Build history of the part. All positions in model axes, mm. Face numbers are marked on the shaded views. Give positions to 0.01 mm unless a question says otherwise; leave off trailing zeros. Order: outer loops, then holes, each group sorted by start corner. A loop starts at its lowest first (then second) coordinate and runs counter-clockwise, first axis right, second up. Notation, with made-up numbers: (-29.75, -12.5) - (18.25, -12.5) arc R20 ccw to (18.25, -4.5) - close; hole circle Ø10 at (18, 79.5). An arc over 180 degrees is marked (long way). One line per item, written item: value.
```python
from build123d import *

# Parameters (mm, degrees)
BOSS_EXTRUDE2_DEPTH = 8
SKETCH2_R           = 3.15
CUT_EXTRUDE1_DEPTH  = 8
BOSS_EXTRUDE4_DEPTH = 2
CUT_EXTRUDE2_DEPTH  = 14
SKETCH5_R           = 2.15
CUT_EXTRUDE3_DEPTH  = 14
SKETCH6_R           = 3.5
CUT_EXTRUDE4_DEPTH  = 2.6
CUT_EXTRUDE5_DEPTH  = 18.5
BOSS_EXTRUDE7_DEPTH = 8
SKETCH9_R           = 3.15
CUT_EXTRUDE6_DEPTH  = 8
CUT_EXTRUDE8_DEPTH  = 8
BOSS_EXTRUDE8_DEPTH = 8
CUT_EXTRUDE9_DEPTH  = 2.5


with BuildPart() as part:
    # Sketch1 → Boss-Extrude2 (new body)
    with BuildSketch(Plane(origin=(0, 0, 0), x_dir=(1, 0, 0), z_dir=(0, 1, 0))):
        Polygon((-36.064195387, 30.19821093), (-36.064195387, 45.055140387), (-24.456215945, 60.508200645), (25.928290152, 75.028423128), (63.192701615, 49.978777876), (57.8600206, 4.654046233), (5.024212079, -12.575443702), (-26.79369062, -0.934399252), align=None)
    extrude(amount=BOSS_EXTRUDE2_DEPTH)

    # Sketch2 → Cut-Extrude1 (cut)
    with BuildSketch(Plane(origin=(0, 8, 0), x_dir=(1, 0, 0), z_dir=(0, 1, 0))):
        with Locations((-0.992606529, 5.023658057)):
            Circle(SKETCH2_R)
        with Locations((-23.973939823, 24.307286348)):
            Circle(SKETCH2_R)
    extrude(amount=-CUT_EXTRUDE1_DEPTH, mode=Mode.SUBTRACT)

    # Sketch3 → Boss-Extrude4 (add)
    with BuildSketch(Plane(origin=(0, 8, 0), x_dir=(1, 0, 0), z_dir=(0, 1, 0))):
        Polygon((-5.747908307, 51.79510143), (2.909877598, 46.790828933), (8.164363719, 55.881504134), (-0.493422186, 60.885776631), align=None)
        Polygon((-2.344608524, 37.700153733), (2.909877598, 46.790828933), (-5.747908307, 51.79510143), (-11.002394429, 42.70442623), align=None)
        Polygon((37.108131922, 27.023952571), (45.765917827, 22.019680074), (51.020403949, 31.110355274), (42.362618044, 36.114627771), align=None)
        Polygon((40.511431705, 12.929004873), (45.765917827, 22.019680074), (37.108131922, 27.023952571), (31.8536458, 17.93327737), align=None)
    extrude(amount=BOSS_EXTRUDE4_DEPTH)

    # Sketch4 → Cut-Extrude2 (cut)
    with BuildSketch(Plane(origin=(0, 8, 0), x_dir=(1, 0, 0), z_dir=(0, 1, 0))):
        Polygon((8.164363719, 55.881504134), (-2.344608524, 37.700153733), (31.8536458, 17.93327737), (42.362618044, 36.114627771), align=None)
    extrude(amount=-CUT_EXTRUDE2_DEPTH, mode=Mode.SUBTRACT)

    # Sketch5 → Cut-Extrude3 (cut)
    with BuildSketch(Plane(origin=(0, 10, 0), x_dir=(1, 0, 0), z_dir=(0, 1, 0))):
        with Locations((-3.921151603, 44.964072229)):
            Circle(SKETCH5_R)
        with Locations((1.083120894, 53.621858134)):
            Circle(SKETCH5_R)
        with Locations((43.939161123, 28.850709275)):
            Circle(SKETCH5_R)
        with Locations((38.934888626, 20.19292337)):
            Circle(SKETCH5_R)
    extrude(amount=-CUT_EXTRUDE3_DEPTH, mode=Mode.SUBTRACT)

    # Sketch6 → Cut-Extrude4 (cut)
    with BuildSketch(Plane.XZ):
        with Locations((43.939161123, -28.850709275)):
            Circle(SKETCH6_R)
        with Locations((38.934888626, -20.19292337)):
            Circle(SKETCH6_R)
        with Locations((1.083120894, -53.621858134)):
            Circle(SKETCH6_R)
        with Locations((-3.921151603, -44.964072229)):
            Circle(SKETCH6_R)
    extrude(amount=-CUT_EXTRUDE4_DEPTH, mode=Mode.SUBTRACT)

    # Sketch7 → Cut-Extrude5 (cut)
    with BuildSketch(Plane(origin=(0, 8, 0), x_dir=(1, 0, 0), z_dir=(0, 1, 0))):
        Polygon((-23.90080129, 101.032848336), (-57.901406204, 20.736967462), (-18.158957139, -32.533824917), (87.924213713, -9.961236853), (85.311975199, 49.315634488), align=None)
        Polygon((-40.820623888, 23.42964982), (-5.371906334, -12.019067733), (42.940552226, -17.400063196), (73.057764711, 41.083606285), (-8.197554073, 82.927487203), align=None, mode=Mode.SUBTRACT)
    extrude(amount=-CUT_EXTRUDE5_DEPTH, mode=Mode.SUBTRACT)

    # Sketch8 → Boss-Extrude7 (add)
    with BuildSketch(Plane(origin=(0, 8, 0), x_dir=(1, 0, 0), z_dir=(0, 1, 0))):
        Polygon((-8.197554073, 82.927487203), (-40.820623888, 23.42964982), (-5.371906334, -12.019067733), (42.940552226, -17.400063196), (73.057764711, 41.083606285), align=None)
        Polygon((7.41963674, 62.005546744), (-9.746922841, 64.747246038), (-32.401642497, 23.42964982), (0, -4.674812176), (46.197479834, 11.841771544), (56.025503799, 35.943618774), align=None, mode=Mode.SUBTRACT)
    extrude(amount=-BOSS_EXTRUDE7_DEPTH)

    # Sketch9 → Cut-Extrude6 (cut)
    with BuildSketch(Plane(origin=(0, 0, 0), x_dir=(-1, 0, 0), z_dir=(0, -1, 0))):
        with Locations((-28.941808693, 3.473889793)):
            Circle(SKETCH9_R)
    extrude(amount=-CUT_EXTRUDE6_DEPTH, mode=Mode.SUBTRACT)

    # Sketch10 → Cut-Extrude8 (cut)
    with BuildSketch(Plane(origin=(0, 8, 0), x_dir=(1, 0, 0), z_dir=(0, 1, 0))):
        Polygon((-51.027907223, 26.499697203), (-18.337970987, 89.979258173), (70.618900133, 64.73001084), (85.862243499, 8.329361683), (41.198193823, -31.646717715), (-23.676019088, -9.814381331), align=None)
        with BuildLine():
            Line((-33.872566493, 31.841833363), (-7.610913822, 63.637460521))
            ThreePointArc((-7.610913822, 63.637460521), (-0.606725689, 67.783190008), (7.431616747, 66.506171896))
            Line((7.431616747, 66.506171896), (48.870452229, 43.677060264))
            ThreePointArc((48.870452229, 43.677060264), (53.514897305, 39.092266426), (55.073012074, 32.754799821))
            Line((55.073012074, 32.754799821), (41.706263242, -9.064889609))
            ThreePointArc((41.706263242, -9.064889609), (33.18888877, -18.343686498), (20.602861854, -17.860296318))
            Line((20.602861854, -17.860296318), (-29.950777497, 7.924950794))
            ThreePointArc((-29.950777497, 7.924950794), (-37.823070784, 18.242703419), (-34.700474084, 30.839465332))
            Line((-34.700474084, 30.839465332), (-33.872566493, 31.841833363))
        make_face(mode=Mode.SUBTRACT)
    extrude(amount=-CUT_EXTRUDE8_DEPTH, mode=Mode.SUBTRACT)

    # Sketch12 → Boss-Extrude8 (add)
    with BuildSketch(Plane(origin=(0, 8, 0), x_dir=(1, 0, 0), z_dir=(0, 1, 0))):
        with BuildLine():
            Line((-34.700474084, 30.839465332), (-23.799416497, 10.878604368))
            Line((-23.799416497, 10.878604368), (16.273254251, -10.775107124))
            Line((16.273254251, -10.775107124), (41.706263242, -9.064889609))
            ThreePointArc((41.706263242, -9.064889609), (33.18888877, -18.343686498), (20.602861854, -17.860296318))
            Line((20.602861854, -17.860296318), (-29.950777497, 7.924950794))
            ThreePointArc((-29.950777497, 7.924950794), (-37.823070784, 18.242703419), (-34.700474084, 30.839465332))
        make_face()
    extrude(amount=-BOSS_EXTRUDE8_DEPTH)

    # Sketch13 → Cut-Extrude9 (cut)
    with BuildSketch(Plane(origin=(0, 10, 0), x_dir=(1, 0, 0), z_dir=(0, 1, 0))):
        Polygon((37.108131922, 27.023952571), (37.608559172, 27.889731161), (43.23612001, 24.636954038), (42.235265511, 22.905396857), (36.607704672, 26.15817398), align=None)
        Polygon((3.410304847, 47.656607524), (-2.217255991, 50.909384647), (-3.21811049, 49.177827466), (2.409450348, 45.925050343), align=None)
    extrude(amount=-CUT_EXTRUDE9_DEPTH, mode=Mode.SUBTRACT)


solid = part.part
```
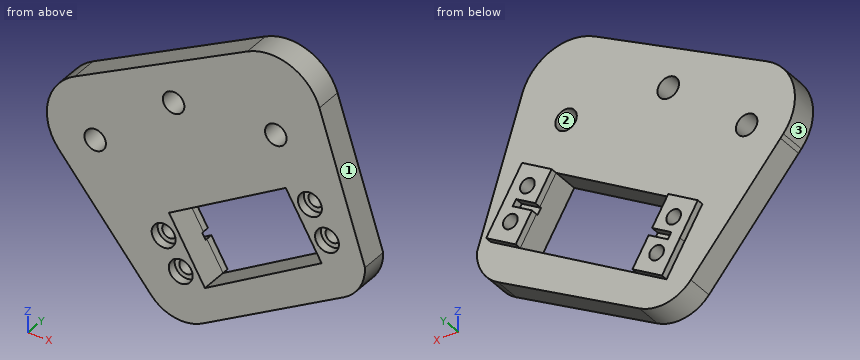
(1) Slice it at B-B, the plane y = 4.5. Count the separate pieces of the cut face and the enclosed holes in it, and give its area (3 significant figures).
Completed:
separate pieces: 1
enclosed holes: 8
area: 4,300 mm²
(2) Slice it at C-C, the plane x = 19.5. Give the cut face in (y, z), and give its area (3 significant figures).
Completed:
outline: (0, -59.86) - (8, -59.86) - (8, -49.33) - (0, -49.33) - close; (0, -25.07) - (8, -25.07) - (8, 17.3) - (0, 17.3) - close
area: 423 mm²
(3) Slice it at D-D, the plane z = 14. Give the cut face in (x, y).
Completed:
outline: (13.03, 0) - (39.02, 0) - (39.02, 8) - (13.03, 8) - close
(4) Slice it at A-A, the plane x = -23.5. Give the cut face in (y, z).
Completed:
outline: (0, -44.4) - (8, -44.4) - (8, -27.42) - (0, -27.42) - close; (0, -21.19) - (8, -21.19) - (8, -4.63) - (0, -4.63) - close
(5) Pin check, flat tips, straight feed: P1, Ø12, axis at x = 32.5, z = -37, coming from the -Y side; P2, Ø3.5, axis at x = -4.5, z = -44.5, coming from the -Y side; P3, Ø3, axis at x = 32, y = 6, coming from the -Z side; P4, Ø1, axis at x = 16, z = -24, coming from the +Y side. Stop position of each tip, or through.
Completed:
P1: y = 0
P2: y = 2.6
P3: z = -53.8
P4: y = 8
(6) Drill centre lines: line 1 (X direction, y = 6.75, z = -29.5); line 2 (Z direction, x = 26.5, y = 2.75); line 3 (X direction, y = 6, z = -29). Where is each one in solid material? Low to high.
Completed:
line 1: -35.69 to 11.84, 38.54 to 41.89, 45.99 to 54.03
line 2: -56 to -45.28, -21.03 to -5.46, -1.48 to 19.47
line 3: -36 to 12.71, 38.25 to 41.79, 46.08 to 53.87
(7) Pull direction X, two halves, no side cores. Call the marked faces 1, 2 and 3: +X half, -X half, draft (parallel to the pull), parting line (faces both ways), or undercut.
Completed:
face 1: +X half
face 2: undercut
face 3: -X half
